The model under review builds one solid part; all positions refer to its coordinate system, in mm. Face numbers are marked on the shaded views. A direction names the side the tool comes from. Coordinates: 2 decimals unless noted, no trailing zeros. Order: outer loops, then holes, each group sorted by start corner. A loop starts at its lowest first (then second) coordinate and runs counter-clockwise, first axis right, second up. Notation, with made-up numbers: (-35, -6.5) -> (-4, -6.5) arc R23 ccw to (-4, 9.5) -> close; hole circle Ø2 at (49, 55). An arc over 180 degrees is marked (long way). Use one line per item in the form item = value.
from build123d import *

# Parameters (mm, degrees)
SKETCH_1_R      = 2.5
EXTRUDE_1_DEPTH = 13.3


with BuildPart() as part:
    # 草图1 → 凸台-拉伸1 (new body)
    with BuildSketch(Plane(origin=(0, 0, 0), x_dir=(0, 0, -1), z_dir=(1, 0, 0))):
        Polygon((-73.839514953, -90.434627318), (-31.839514953, -90.434627318), (-31.839514953, -84.434627318), (-43.839514953, -84.434627318), (-43.839514953, -58.434627318), (-61.839514953, -58.434627318), (-61.839514953, -84.434627318), (-73.839514953, -84.434627318), align=None)
        with Locations((-52.839514953, -70.934627318)):
            Circle(SKETCH_1_R, mode=Mode.SUBTRACT)
    extrude(amount=EXTRUDE_1_DEPTH)


solid = part.part
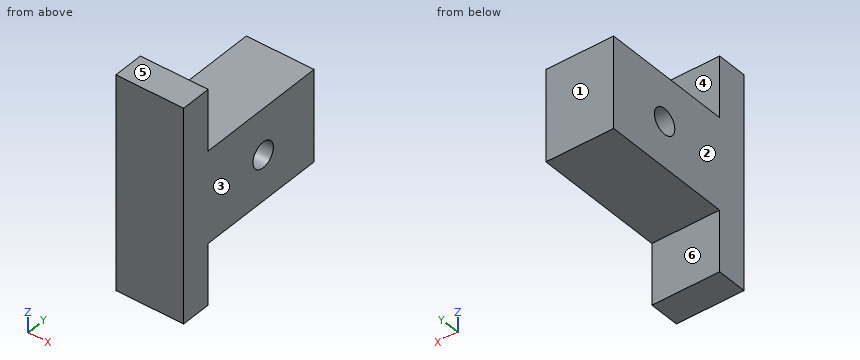
Item 1: We need section B-B (x = 11.5). Write out the cut boundary in (y, z).
Results found:
outline = (-90.43, 31.84) -> (-84.43, 31.84) -> (-84.43, 43.84) -> (-58.43, 43.84) -> (-58.43, 61.84) -> (-84.43, 61.84) -> (-84.43, 73.84) -> (-90.43, 73.84) -> close; hole circle Ø5 at (-70.93, 52.84)
Item 2: We need section A-A (z = 51). Write out the cut boundary in (x, y).
Results found:
outline = (0, -90.43) -> (13.3, -90.43) -> (13.3, -72.63) -> (0, -72.63) -> close; (0, -69.24) -> (13.3, -69.24) -> (13.3, -58.43) -> (0, -58.43) -> close
Item 3: Draft analysis for pull direction X (two halves, no side actions). For the marked faces 1, 2 and 3, state which applies: released by +X, released by -X, zero draft, split by the parting line, or undercut.
Results found:
face_1 = zero draft
face_2 = released by -X
face_3 = released by +X
Item 4: To check wall thickness, follow L1, parallel to Z at x = 3.25, y = -73.5; L2, parallel to Y at x = 4.5, z = 64.5; L3, parallel to Z at x = 1.25, y = -70. State the ranges of each line that lie inside material, in increasing order. Write a range as from..to.
Results found:
L1 = 43.84..61.84
L2 = -90.43..-84.43
L3 = 43.84..50.52, 55.16..61.84
Item 5: We need section C-C (y = -66). Write out the cut boundary in (x, z).
Results found:
outline = (0, 43.84) -> (13.3, 43.84) -> (13.3, 61.84) -> (0, 61.84) -> close
Item 6: Tool access review of the marked faces 4, 5 and 6: name each direction out of +Z, -Z, +X, -X, +Y, -Y from which nothing blocks a thin tool from reaching the whole face with its end or side.
Results found:
face_4 = +Z, +X, -X, +Y
face_5 = +Z, +X, -X, +Y, -Y
face_6 = -Z, +X, -X, +Y
Item 7: We need section D-D (z = 63.5). Write out the cut boundary in (x, y).
Results found:
outline = (0, -90.43) -> (13.3, -90.43) -> (13.3, -84.43) -> (0, -84.43) -> close
Item 8: Clearance check with flat-ended pins moving along their axes: pin 1 (3.5 mm diameter, centred on x = 7, z = 36, fed in from +Y); pin 2 (4 mm diameter, centred on x = 4, y = -68, fed in from -Z); pin 3 (6.5 mm diameter, centred on y = -70.93, z = 52.84, fed in from -X). State where each tip first meets the part, or that it passes through.
Results found:
pin_1 = -84.43
pin_2 = 43.84
pin_3 = 0
